```python
from build123d import *

# Parameters (mm, degrees)
EXTRUDE_1_DEPTH     = 2.9
SKETCH_2_R          = 3.5
EXTRUDE_2_DEPTH     = 2.1
SKETCH_3_R          = 2
CUT_EXTRUDE_1_DEPTH = 8.320063752
FILLET_1_R          = 1.2


with BuildPart() as part:
    # 草图1 → 凸台-拉伸1 (new body)
    with BuildSketch(Plane.XY):
        Polygon((3.5, -2.020725942), (3.5, 2.020725942), (0, 4.041451884), (-3.5, 2.020725942), (-3.5, -2.020725942), (0, -4.041451884), align=None)
    extrude(amount=EXTRUDE_1_DEPTH)

    # 草图2 → 凸台-拉伸2 (add)
    with BuildSketch(Plane.XY.offset(2.9)):
        Circle(SKETCH_2_R)
    extrude(amount=EXTRUDE_2_DEPTH)

    # 草图3 → 切除-拉伸1 (cut, through all)
    with BuildSketch(Plane.XY.offset(5)):
        Circle(SKETCH_3_R)
    extrude(amount=-CUT_EXTRUDE_1_DEPTH, mode=Mode.SUBTRACT)

    # 圆角1
    fillet_1_edges = [part.edges().sort_by_distance(p)[0] for p in [
        (-3.5, 0, 5),
    ]]
    fillet(fillet_1_edges, radius=FILLET_1_R)


solid = part.part
```
CAD build for the part. Positions are in the model's coordinates, mm. A direction names the side the tool comes from. Round coordinates to 2 decimals unless told otherwise and drop trailing zeros. Loops run counter-clockwise (first coordinate to the right, second up) from the corner with the lowest first, then second, coordinate; pieces in that order, holes last. Notation, with made-up numbers: M -19,0.5 L -6,0.5 A16 ccw -6,11.5 Z; hole C -22,59 d5. An arc over 180 degrees is marked long. Use a Markdown table: item, result. Add a question column.
(1) Which spindle directions (+Z, -Z, +X, -X, +Y, -Y) get a long thin tool onto all of the face, cutting with end or side? Do faces 4 (the face through (3.233, -1.341, 3.344)), 5 (the face through (3.2, -1.8, 2.9)), 6 (the face through (-3.15, -1.85, 2.9)), 7 (the face through (0, -3.7, 2.9)), 8 (the face through (-3.15, 1.86, 2.9)). Say none if no direction does.
(2) Cut at B-B (y = 3.75). Give the cut face in (x, z).
(3) Drill centre lines: line 1 (Y direction, x = 0, z = 3.3); line 2 (X direction, y = 1, z = 3.45); line 3 (X direction, y = 1.75, z = 1.7). Where is each one in solid material? Low to high.
(4) Cut at A-A (z = 2.3). Give the cut face in (x, y).
(5) Cut at C-C (z = 3.7). Give the cut face in (x, y).
(6) Pull direction Y, two halves, no side cores. Call faces 1 (the face through (-1.8, -3, 1.4)), 2 (the face through (-3.5, 0, 1)), 3 (the face through (0, -2, 3)): +Y half, -Y half, draft (parallel to the pull), parting line (faces both ways), or undercut.
(7) Flat gauge pins, fed straight in: pin 1 (0.8 mm diameter, centred on x = 0.5, y = 3.5, fed in from +Z); pin 2 (3 mm diameter, centred on x = 0, y = 0, fed in from -Z); pin 3 (1.5 mm diameter, centred on x = -0.5, z = 1, fed in from +Y); pin 4 (0.5 mm diameter, centred on x = -0.5, y = -3.5, fed in from +Z). Where does each tip first touch, or does it go through?
Geometry says:
| question | item | result |
|---|---|---|
| 1 | face 4 | +Z |
| 1 | face 5 | +Z, +X, -Y |
| 1 | face 6 | +Z, -X, -Y |
| 1 | face 7 | +Z, -Y |
| 1 | face 8 | +Z, -X, +Y |
| 2 | outline | M -0.5,0 L 0.5,0 L 0.5,2.9 L -0.5,2.9 Z |
| 3 | line 1 | y = -3.5 to -2, 2 to 3.5 |
| 3 | line 2 | x = -3.35 to -1.73, 1.73 to 3.35 |
| 3 | line 3 | x = -3.5 to -0.97, 0.97 to 3.5 |
| 4 | outline | M -3.5,-2.02 L 0,-4.04 L 3.5,-2.02 L 3.5,2.02 L 0,4.04 L -3.5,2.02 Z; hole C 0,0 d4 |
| 5 | outline | C 0,0 d7; hole C 0,0 d4 |
| 6 | face 1 | -Y half |
| 6 | face 2 | draft |
| 6 | face 3 | undercut |
| 7 | pin 1 | stops at z = 4.66 |
| 7 | pin 2 | passes through |
| 7 | pin 3 | stops at y = 4.04 |
| 7 | pin 4 | stops at z = 4.48 |
